Input: part model. Units: mm. Frame: model coordinates. A direction names the side the tool comes from. Round coordinates to 2 decimals unless told otherwise and drop trailing zeros. Loops run counter-clockwise (first coordinate to the right, second up) from the corner with the lowest first, then second, coordinate; pieces in that order, holes last. Notation, with made-up numbers: M 6.5,-30.5 L 63.5,-30.5 A14 ccw 63.5,-24.5 Z; hole C -15.5,-3 d10. An arc over 180 degrees is marked long. Put each result on its own line as item: value. Start each with the question number.
1) Line query: probe 1 along X at (y, z) = (3.5, -18.5); probe 2 along Z at (x, y) = (71, -6); probe 3 along Y at (x, z) = (78, 0). Output: solid intervals per line, ascending.
2) Reachability of faces 1 (the face through (83.96, 2.17, 9.76)), 2 (the face through (100, 0, 0)), 3 (the face through (20, -6, 6)) from +Z, -Z, +X, -X, +Y, -Y: full face, straight path, thin tool, end or side. Return the list, or none.
3) Pin query (flat end, axial travel): pin 1 (12 mm diameter, centred on x = 56.5, z = 2, fed in from -Y); pin 2 (8 mm diameter, centred on x = 38, z = 15.5, fed in from +Y); pin 3 (5 mm diameter, centred on x = 49, z = -3, fed in from +Y); pin 4 (10 mm diameter, centred on x = 44, y = 7.5, fed in from -Z). Return the tip coordinate at first contact, or that it passes through.
4) Section A-A on x = 11.5. Output: boundary loops of the cut face in (y, z), plus the area to 3 significant figures.
Autodesk Inventor part; units mm, degrees
ref_plane "YZ Plane" through (0, 0, 0) normal (1, 0, 0) x (0, 1, 0)
ref_plane "XZ Plane" through (0, 0, 0) normal (0, 1, 0) x (-1, 0, 0)
ref_plane "XY Plane" through (0, 0, 0) normal (0, 0, 1) x (1, 0, 0)
sketch "Sketch1" plane through (0, 0, 0) normal (0, 0, 1) x (1, 0, 0)
  line L0 (100, 10) -> (100, 0)
  line L1 (50.009, 15) -> (20.009, 15)
  line L2 (20.009, 15) -> (20.009, 15)
  line L3 (20.009, 15) -> (20, 15)
  line L4 (20, 15) -> (20, 8)
  line L5 (20, 8) -> (0, 8)
  line L6 (0, 8) -> (0, 0)
  line L7 (50.009, 15) -> (50.009, 22.5)
  line L8 (50.009, 22.5) -> (65.009, 22.5)
  line L9 (65.009, 22.5) -> (65.009, 10)
  line L10 (65.009, 10) -> (100, 10)
  line L11 (100, 10) -> (100, 10)
  line L12 (0, 0) -> (100, 0)
  dimension "d0" = 100
  dimension "d5" = 20
  dimension "d6" = 30
  dimension "d7" = 20
  dimension "d8" = 45
  dimension "d9" = 30
  dimension "d10" = 16
  dimension "d11" = 15
revolve "Revolution1" add sketch "Sketch1" angle 360 mid plane about axis through (0, 0, 0) along (1, 0, 0)
chamfer "Chamfer1" distance 1.5 angle 45 1 edges at (100, 10, 0)
fillet "Fillet1" radius 4 1 edges at (65.009, 10, 0)
fillet "Fillet2" radius 2 1 edges at (65.009, 22.5, 0)
chamfer "Chamfer2" distance 2 angle 45 1 edges at (20, 15, 0)
chamfer "Chamfer3" distance 1 angle 45 1 edges at (0, 8, 0)
Geometry results:
1. probe 1: x = 50.01 to 65.01
1. probe 2: z = -8 to 8
1. probe 3: y = -10 to 10
2. face 1: +X
2. face 2: +Z, -Z, +X, +Y, -Y
2. face 3: -X
3. pin 1: stops at y = -22.5
3. pin 2: stops at y = 9.63
3. pin 3: stops at y = 22.49
3. pin 4: stops at z = -14.79
4. outline: C 0,0 d16
4. area: 201 mm²
